```python
from build123d import *

# Parameters (mm, degrees)
SKETCH1_R           = 50
SKETCH1_R_2         = 40
BOSS_EXTRUDE1_DEPTH = 10
BOSS_EXTRUDE3_DEPTH = 5
FILLET1_R           = 32
FILLET2_R           = 4
CHAMFER1_SIZE       = 1
FILLET3_R           = 1.5
SKETCH2_R           = 8
SKETCH2_R_2         = 3
BOSS_EXTRUDE4_DEPTH = 18
CHAMFER2_SIZE       = 1
SKETCH3_R           = 1.6
CUT_EXTRUDE1_DEPTH  = 10


with BuildPart() as part:
    # Sketch1 → Boss-Extrude1 (new body)
    with BuildSketch(Plane.XY):
        Circle(SKETCH1_R)
        Circle(SKETCH1_R_2, mode=Mode.SUBTRACT)
    extrude(amount=BOSS_EXTRUDE1_DEPTH)

    # Sketch1<5> → Boss-Extrude3 (add)
    with BuildSketch(Plane.XY):
        with BuildLine():
            ThreePointArc((4, 39.799497484), (0, 40), (-4, 39.799497484))
            Line((-4, 39.799497484), (-4, 2.309401077))
            Line((-4, 2.309401077), (-36.467375879, -16.435647127))
            ThreePointArc((-36.467375879, -16.435647127), (-34.641016151, -20), (-32.467375879, -23.363850357))
            Line((-32.467375879, -23.363850357), (0, -4.618802154))
            Line((0, -4.618802154), (32.467375879, -23.363850357))
            ThreePointArc((32.467375879, -23.363850357), (34.641016151, -20), (36.467375879, -16.435647127))
            Line((36.467375879, -16.435647127), (4, 2.309401077))
            Line((4, 2.309401077), (4, 39.799497484))
        make_face()
    extrude(amount=BOSS_EXTRUDE3_DEPTH)

    # Fillet1
    fillet1_edges = [part.edges().sort_by_distance(p)[0] for p in [
        (-4, 2.309401077, 2.5),
        (0, -4.618802154, 2.5),
        (4, 2.309401077, 2.5),
    ]]
    fillet(fillet1_edges, radius=FILLET1_R)

    # Fillet2
    fillet2_edges = [part.edges().sort_by_distance(p)[0] for p in [
        (-36.467375879, -16.435647127, 2.5),
        (-32.467375879, -23.363850357, 2.5),
        (32.467375879, -23.363850357, 2.5),
        (36.467375879, -16.435647127, 2.5),
        (4, 39.799497484, 2.5),
        (-4, 39.799497484, 2.5),
    ]]
    fillet(fillet2_edges, radius=FILLET2_R)

    # Chamfer1
    chamfer1_edges = [part.edges().sort_by_distance(p)[0] for p in [
        (0, -9.569219382, 0),
        (-8.287187079, 4.784609691, 0),
        (8.287187079, 4.784609691, 0),
        (26.198684154, -10.507015195, 0),
        (31.269438399, 24.944382578, 0),
        (0, -40, 0),
        (-34.641016151, 20, 0),
        (22.198684154, -17.435218425, 0),
        (-26.198684154, -10.507015195, 0),
        (-22.198684154, -17.435218425, 0),
        (-4, 27.94223362, 0),
        (4, 27.94223362, 0),
        (35.85816198, -14.345444364, 0),
        (30.352600238, -23.881357026, 0),
        (-35.85816198, -14.345444364, 0),
        (-30.352600238, -23.881357026, 0),
        (-5.505561742, 38.226801389, 0),
        (5.505561742, 38.226801389, 0),
    ]]
    chamfer(chamfer1_edges, length=CHAMFER1_SIZE)

    # Fillet3
    fillet3_edges = [part.edges().sort_by_distance(p)[0] for p in [
        (-50, 0, 10),
        (-50, 0, 0),
    ]]
    fillet(fillet3_edges, radius=FILLET3_R)

    # Sketch2 → Boss-Extrude4 (add)
    with BuildSketch(Plane.XY.offset(5)):
        Circle(SKETCH2_R)
        Circle(SKETCH2_R_2, mode=Mode.SUBTRACT)
    extrude(amount=BOSS_EXTRUDE4_DEPTH)

    # Chamfer2
    chamfer2_edges = [part.edges().sort_by_distance(p)[0] for p in [
        (-8, 0, 23),
        (-8, 0, 5),
    ]]
    chamfer(chamfer2_edges, length=CHAMFER2_SIZE)

    # Sketch3 → Cut-Extrude1 (cut)
    with BuildSketch(Plane(origin=(0, 0, 0), x_dir=(0, 0, -1), z_dir=(1, 0, 0))):
        with Locations((-19, 0)):
            Circle(SKETCH3_R)
        with Locations((-13, 0)):
            Circle(SKETCH3_R)
    extrude(amount=-CUT_EXTRUDE1_DEPTH, mode=Mode.SUBTRACT)


solid = part.part
```
Input: part model. Units: mm. Frame: model coordinates. A direction names the side the tool comes from. Give positions to 0.01 mm unless a question says otherwise; leave off trailing zeros. Order: outer loops, then holes, each group sorted by start corner. A loop starts at its lowest first (then second) coordinate and runs counter-clockwise, first axis right, second up. Notation, with made-up numbers: (2.25, 49.25) - (29.25, 49.25) arc R25 ccw to (29.25, 73.25) - close; hole circle Ø8 at (-20, 40.5). An arc over 180 degrees is marked (long way). One line per item, written item: value.
1. Cut plane A-A, the plane x = 0. Output: boundary loops of the cut face in (y, z).
Determined:
outline: (-50, 1.5) arc R1.5 ccw to (-48.5, 0) - (-41, 0) - (-40, 1) - (-40, 10) - (-48.5, 10) arc R1.5 ccw to (-50, 8.5) - close; (-9.57, 1) - (-8.57, 0) - (48.5, 0) arc R1.5 ccw to (50, 1.5) - (50, 8.5) arc R1.5 ccw to (48.5, 10) - (40, 10) - (40, 5) - (9, 5) - (8, 6) - (8, 22) - (7, 23) - (3, 23) - (3, 5) - (-3, 5) - (-3, 23) - (-7, 23) - (-8, 22) - (-8, 6) - (-9, 5) - (-9.57, 5) - close
2. Line query: probe 1 along Y at (x, z) = (0, 5.75); probe 2 along X at (y, z) = (15, 4); probe 3 along X at (y, z) = (7.5, 3.25). Output: solid intervals per line, ascending.
Determined:
probe 1: -50 to -40, -8.25 to -3, 3 to 8.25, 40 to 50
probe 2: -47.7 to -37.08, -4.53 to 4.53, 37.08 to 47.7
probe 3: -49.43 to -39.29, -6.89 to 6.89, 39.29 to 49.43
3. Cut plane B-B, the plane z = 3.75. Output: boundary loops of the cut face in (x, y).
Determined:
outline: circle Ø100 at (0, 0); hole (-38.22, -11.8) arc R4 ccw to (-32.4, -14.09) - (-20, -6.93) arc R32 ccw to (-4, 20.78) - (-4, 35.1) arc R4 ccw to (-8.89, 39) arc R40 ccw to start; hole (-29.33, -27.2) arc R40 ccw to (29.33, -27.2) arc R4 ccw to (28.4, -21.01) - (16, -13.86) arc R32 ccw to (-16, -13.86) - (-28.4, -21.01) arc R4 ccw to start; hole (4, 20.78) arc R32 ccw to (20, -6.93) - (32.4, -14.09) arc R4 ccw to (38.22, -11.8) arc R40 ccw to (8.89, 39) arc R4 ccw to (4, 35.1) - close
4. Cut plane C-C, the plane y = 0. Give the number of separate pieces and of enclosed holes in the cut face, and give its area (3 significant figures).
Determined:
separate pieces: 5
enclosed holes: 0
area: 460 mm2
5. Pin query (flat end, axial travel): pin 1 Ø1.8 at (x, y) = (0, -0.5) entering from +Z; pin 2 Ø12 at (x, z) = (-5, 7.5) entering from +Y; pin 3 Ø3 at (y, z) = (25.5, 2.5) entering from -X; pin 4 Ø6 at (x, z) = (-24, 14.5) entering from +Y. Return the tip coordinate at first contact, or that it passes through.
Determined:
pin 1: z = 5
pin 2: y = 50
pin 3: x = -43.86
pin 4: through
6. Reachability of faces 3 (the face through (-0.23, -9.57, 3.03)), 4 (the face through (1, -3, 23)), 5 (the face through (7.39, -3.06, 13.89)), 6 (the face through (8.03, 4.91, 0.84)), 7 (the face through (-5.231, 1.586, 19.208)) from +Z, -Z, +X, -X, +Y, -Y: full face, straight path, thin tool, end or side. Return the list, or none.
Determined:
face 3: +Z, -Z
face 4: +Z, +X, -X, +Y, -Y
face 5: +Z
face 6: -Z
face 7: -X
7. Draft query along Y for faces 1 (the face through (26.29, -10.56, 2.97)), 2 (the face through (-1, 1, 0)). Return one class per face: released by +Y, released by -Y, zero draft, split by the parting line, or undercut.
Determined:
face 1: undercut
face 2: zero draft
